Autodesk Inventor part; units mm, degrees
ref_plane "YZ Plane" through (0, 0, 0) normal (1, 0, 0) x (0, 1, 0)
ref_plane "XZ Plane" through (0, 0, 0) normal (0, 1, 0) x (-1, 0, 0)
ref_plane "XY Plane" through (0, 0, 0) normal (0, 0, 1) x (1, 0, 0)
sketch "Sketch1" plane through (0, 0, 0) normal (0, 1, 0) x (-1, 0, 0)
  circle A0 centre (0, 0) radius 8.25
  dimension "d0" = 16.5
extrude "Extrusion1" add sketch "Sketch1" along normal blind 7.3
sketch "Sketch3" plane through (0, 7.3, 0) normal (0, 1, 0) x (1, 0, 0)
  line L0 (-7.65, 3) -> (7.65, 3)
  line L1 (7.65, 3) -> (7.65, 15.1)
  line L2 (7.65, 15.1) -> (-7.65, 15.1)
  line L3 (-7.65, 15.1) -> (-7.65, 3)
  point P0 (0, 0)
  dimension "d3" = 15.3
  dimension "d4" = 3
  dimension "d5" = 7.65
  dimension "d6" = 12.1
extrude "Extrusion2" add sketch "Sketch3" against normal blind 1.3
sketch "Sketch4" plane through (0, 7.3, 0) normal (0, 1, 0) x (1, 0, 0)
  circle A0 centre (0, 0) radius 8.25
  dimension "d9" = 16.5
extrude "Extrusion3" add sketch "Sketch4" along normal blind 2
sketch "Sketch5" plane through (0, 9.3, 0) normal (0, 1, 0) x (1, 0, 0)
  circle A0 centre (0, 0) radius 2.9
  dimension "d12" = 5.8
extrude "Extrusion4" add sketch "Sketch5" along normal blind 21
properties part number "Potentiometer_Model"
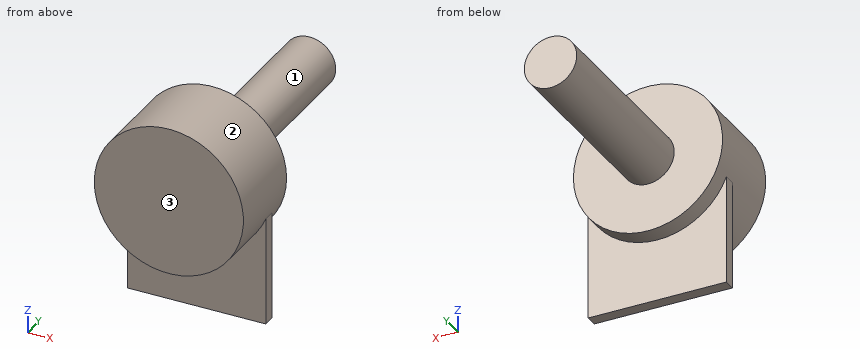
Model file for the job. Use its own axes, mm. Face numbers are marked on the shaded views. A direction names the side the tool comes from. Coordinates: 2 decimals unless noted, no trailing zeros. Order: outer loops, then holes, each group sorted by start corner. A loop starts at its lowest first (then second) coordinate and runs counter-clockwise, first axis right, second up. Notation, with made-up numbers: (69, 80.5) - (84, 80.5) arc R5 cw to (84, 86.5) - close; hole circle Ø1 at (13.25, -14). An arc over 180 degrees is marked (long way). Return JSON: item names as keys, results as strings. Group by question number.
1) Tool access for the marked faces 1, 2 and 3: list every direction of +Z, -Z, +X, -X, +Y, -Y with a clear straight run to the whole face (end or side of a thin tool).
2) Probe line 1 (Y direction, x = 4.5, z = -4.5); line 2 (Y direction, x = 3.75, z = -12.5); line 3 (X direction, y = 7, z = -0.25). List the from-to ranges inside material, lowest first. Write a range as from..to.
3) Flat gauge pins, fed straight in: P1, Ø5, axis at x = 0.5, y = 13.5, coming from the -Z side; P2, Ø3.5, axis at x = -1.5, z = -11.5, coming from the -Y side; P3, Ø4, axis at y = 19, z = -4.5, coming from the -X side; P4, Ø8, axis at x = 1.5, z = 5.5, coming from the +Y side. Where does each tip first touch, or does it go through?
4) Saw through at A-A, the plane z = -11. Write the cut outline in (x, y).
5) Saw through at B-B, the plane y = 10. Write the cut outline in (x, z).
Values found:
{
 "1": {"face 1": "+Y", "face 2": "none", "face 3": "+Z, -Z, +X, -X, -Y"},
 "2": {"line 1": "y = 0..9.3", "line 2": "y = 6..7.3", "line 3": "x = -8.25..8.25"},
 "3": {"P1": "stops at z = -2.9", "P2": "stops at y = 6", "P3": "stops at x = -1.47", "P4": "stops at y = 30.3"},
 "4": {"outline": "(-7.65, 6) - (7.65, 6) - (7.65, 7.3) - (-7.65, 7.3) - close"},
 "5": {"outline": "circle Ø5.8 at (0, 0)"}
}
